Geometry: see drawing. Coordinates: mm, zero at the bounding-box minimum. A direction names the side the tool comes from. Give positions to 0.01 mm unless a question says otherwise; leave off trailing zeros. Write each loop counter-clockwise with the first axis right and the second up, starting at its lowest first coordinate (ties: lowest second). Pieces come first, ordered by that corner, then holes. Notation, with made-up numbers: (-22, 46) - (25, 46) arc R21 ccw to (25, 59) - close; hole circle Ø5 at (2.5, 19.25). An arc over 180 degrees is marked (long way). One line per question, with ' | ' between items. Start each with the question number.
(1) Pin query (flat end, axial travel): pin 1 (1.5 mm diameter, centred on x = 303.5, z = 223.5, fed in from +Y). Return the tip coordinate at first contact, or that it passes through.
(2) Section A-A, the plane z = 161.5. Return loops of the section in (x, y), plus the area to 4 significant figures.
(3) Draft query along X for the marked faces 3, 4 and 5. Return one class per face: +X half, -X half, draft (parallel to the pull), parting line (faces both ways), or undercut.
(4) Section B-B, the plane y = 14. Return loops of the section in (x, z).
(5) Ray query, line 1 (X direction, y = 37, z = 223.75); line 2 (Z direction, x = 303.75, y = 39.5); line 3 (X direction, y = 22.5, z = 261.5). Return the intervals inside material, ascending. Write a range as [from, to].
(6) Access query for the marked faces 1 and 2. Directions: +Z, -Z, +X, -X, +Y, -Y. A direction counts if a zero-diameter tool reaches every point of the face in a straight line with its end or side. Return the directions, or none.
(7) Section C-C, the plane x = 51. Return loops of the section in (y, z).
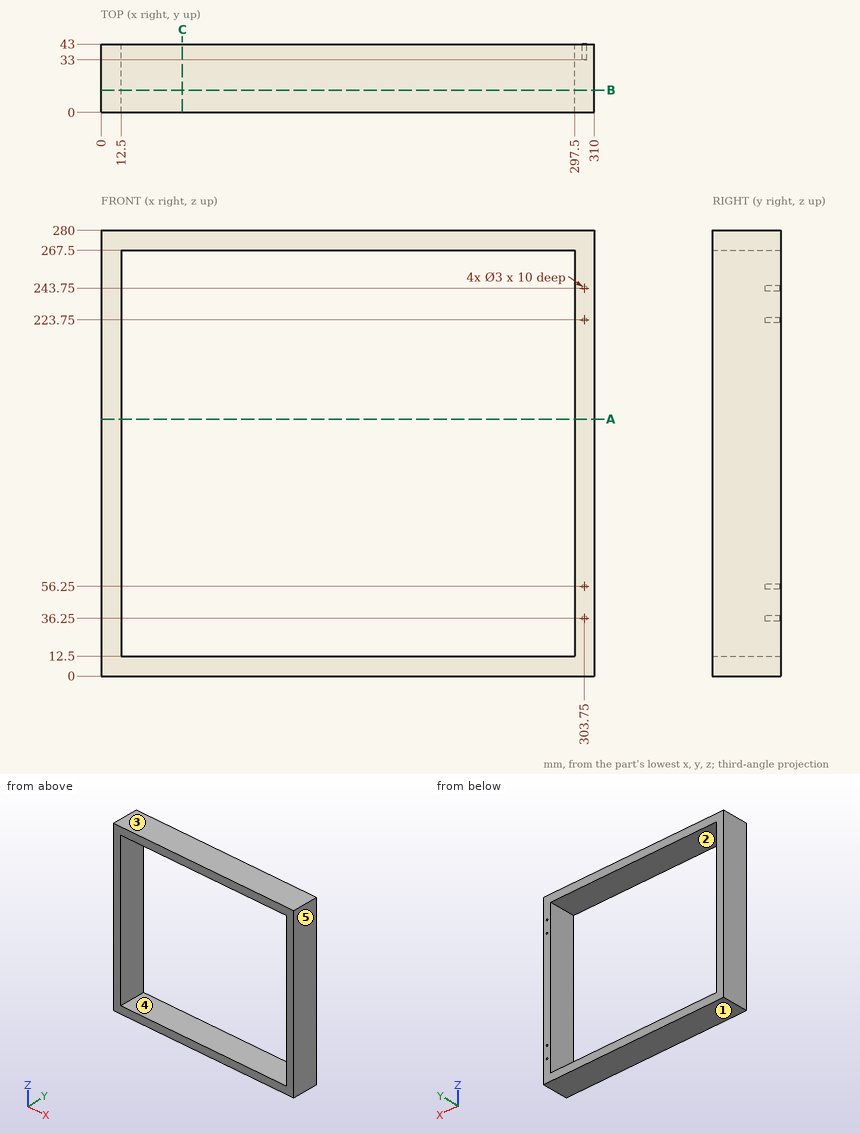
Check sheet entries:
1) pin 1: y = 33
2) outline: (0, 0) - (12.5, 0) - (12.5, 43) - (0, 43) - close; (297.5, 0) - (310, 0) - (310, 43) - (297.5, 43) - close | area: 1,075 mm²
3) face 3: draft | face 4: undercut | face 5: +X half
4) outline: (0, 0) - (310, 0) - (310, 280) - (0, 280) - close; hole (12.5, 12.5) - (297.5, 12.5) - (297.5, 267.5) - (12.5, 267.5) - close
5) line 1: [0, 12.5], [297.5, 302.25], [305.25, 310] | line 2: [0, 34.75], [37.75, 54.75], [57.75, 222.25], [225.25, 242.25], [245.25, 280] | line 3: [0, 12.5], [297.5, 310]
6) face 1: -Z, +X, -X, +Y, -Y | face 2: +Y, -Y
7) outline: (0, 0) - (43, 0) - (43, 12.5) - (0, 12.5) - close; (0, 267.5) - (43, 267.5) - (43, 280) - (0, 280) - close
